from build123d import *

# Parameters (mm, degrees)
F3_DEPTH = 3.175
F5_DEPTH = 2.54
F6_R     = 2.539


# Not quite as in the source:
# - a fillet or chamfer is up to 0.001 mm smaller than in the source, because OpenCascade refuses the exact size


with BuildPart() as f1:
    # F0 (on Right) → F1 (revolve)
    with BuildSketch(Plane.YZ):
        with BuildLine():
            Line((0, 6.35), (0, 0))
            Line((0, 0), (63.5, 0))
            Line((63.5, 0), (63.5, 3.81))
            ThreePointArc((63.5, 3.81), (31.7753898481, 5.714746203), (0, 6.35))
        make_face()
    revolve(axis=Axis((0, 0, 3.175), (0, 0, 1)))

    # F2 (on Front) → F3 (join, symmetric)
    with BuildSketch(Plane.XZ):
        with BuildLine():
            Line((-63.246, 0), (-50.546, 0))
            Line((-50.546, 0), (-50.546, 128.6024183169))
            ThreePointArc((-50.546, 128.6024183169), (-36.3147984428, 168.6628164677), (0, 190.7670697195))
            ThreePointArc((0, 190.7670697195), (4.9210651403, 198.2789348597), (-2.5908, 203.2))
            ThreePointArc((-2.5908, 203.2), (-46.1685581314, 176.6748960979), (-63.246, 128.6024183169))
            Line((-63.246, 128.6024183169), (-63.246, 0))
        make_face()
    extrude(amount=F3_DEPTH, both=True)

    # F4 (on Front) → F5 (join, symmetric)
    with BuildSketch(Plane.XZ):
        with BuildLine():
            Line((0.9183558658, 171.6801895282), (-1.2954, 196.9835348597))
            Line((-1.2954, 196.9835348597), (-6.3496308803, 196.4671948838))
            Line((-6.3496308803, 196.4671948838), (-4.1423132005, 171.2374383551))
            ThreePointArc((-4.1423132005, 171.2374383551), (9.8943909909, 158.4855183155), (23.7102105401, 171.4764251136))
            Line((23.7102105401, 171.4764251136), (18.6384196387, 171.7741938758))
            ThreePointArc((18.6384196387, 171.7741938758), (9.8216872219, 163.5651291728), (0.9183558658, 171.6801895282))
        make_face()
    extrude(amount=F5_DEPTH, both=True)

    # F6 (radius 2.54 in the source; OpenCascade refuses exactly that, so slightly less here)
    f6_edges = [f1.edges().sort_by_distance(p)[0] for p in [
        (0.090338, -2.54, 181.144481),
        (0.090338, 2.54, 181.144481),
        (9.821687, -2.54, 163.565129),
        (9.894391, -2.54, 158.485518),
        (-4.932181, -2.54, 180.265666),
        (9.894391, 2.54, 158.485518),
        (-4.932181, 2.54, 180.265666),
        (9.821687, 2.54, 163.565129),
    ]]
    fillet(f6_edges, radius=F6_R)


solid = f1.part
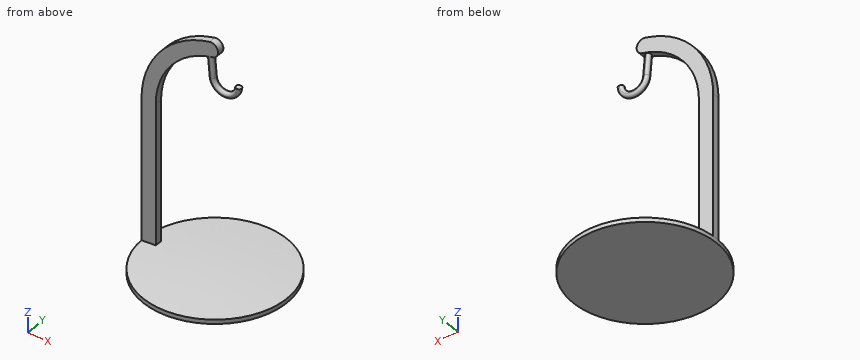
Work out the finished part from the listing and answer in its coordinate system (mm). Coordinates: 2 decimals unless noted, no trailing zeros. Loops run counter-clockwise (first coordinate to the right, second up) from the corner with the lowest first, then second, coordinate; pieces in that order, holes last. Notation, with made-up numbers: M 16,-26 L 73,-26 A4 cw 73,-21 Z; hole C 65.25,-27.5 d6. An arc over 180 degrees is marked long. Answer in a Markdown table with one row per item. Add a question column.
1. Consider L1, parallel to X at y = 1.5, z = 181; L2, parallel to Z at x = 44.5, y = -7.5; L3, parallel to Z at x = 21.5, y = 8. Determine where each line is inside the solid, lowest interval first.
2. Find section B-B, the plane z = 41.5. Write down the section's boundary in (x, y) (3 decimals).
3. Flat-ended cylindrical pins translate along their axes: P1, Ø7, axis at y = 0.5, z = 37, coming from the -X side; P2, Ø3, axis at y = -1.5, z = 92, coming from the +X side. Find the tip coordinate at first contact, or state that the pin passes through.
4. Find section A-A, the plane x = -44. Write down the section's boundary in (y, z) (3 decimals).
5. Find section C-C, the plane y = -12.5. Write down the section's boundary in (x, z).
Reported:
| question | item | result |
|---|---|---|
| 1 | L1 | x = -42.37 to -22.92, -4.5 to -0.39 |
| 1 | L2 | z = 0 to 5.07 |
| 1 | L3 | z = 0 to 6.02 |
| 2 | outline | M -63.246,-3.175 L -50.546,-3.175 L -50.546,3.175 L -63.246,3.175 Z |
| 3 | P1 | stops at x = -63.25 |
| 3 | P2 | stops at x = -50.55 |
| 4 | outline | M -45.785,0 L 45.785,0 L 45.785,3.81 A793.801 ccw -45.785,3.81 Z; M -3.175,156.683 L 3.175,156.683 L 3.175,179.225 L -3.175,179.225 Z |
| 5 | outline | M -62.26,0 L 62.26,0 L 62.26,3.81 A794.92 ccw -62.26,3.81 Z |
